Check sheet for the drawn part. Datum: minimum x, y, z corner. Units: mm. Round coordinates to 2 decimals unless told otherwise and drop trailing zeros. Write each loop counter-clockwise with the first axis right and the second up, starting at its lowest first coordinate (ties: lowest second). Pieces come first, ordered by that corner, then holes. Notation, with made-up numbers: (6.5, -24) -> (37.5, -24) arc R19 cw to (37.5, -19) -> close; hole circle Ø10 at (23.5, 36). An arc over 180 degrees is marked (long way). One line per item, written item: value.
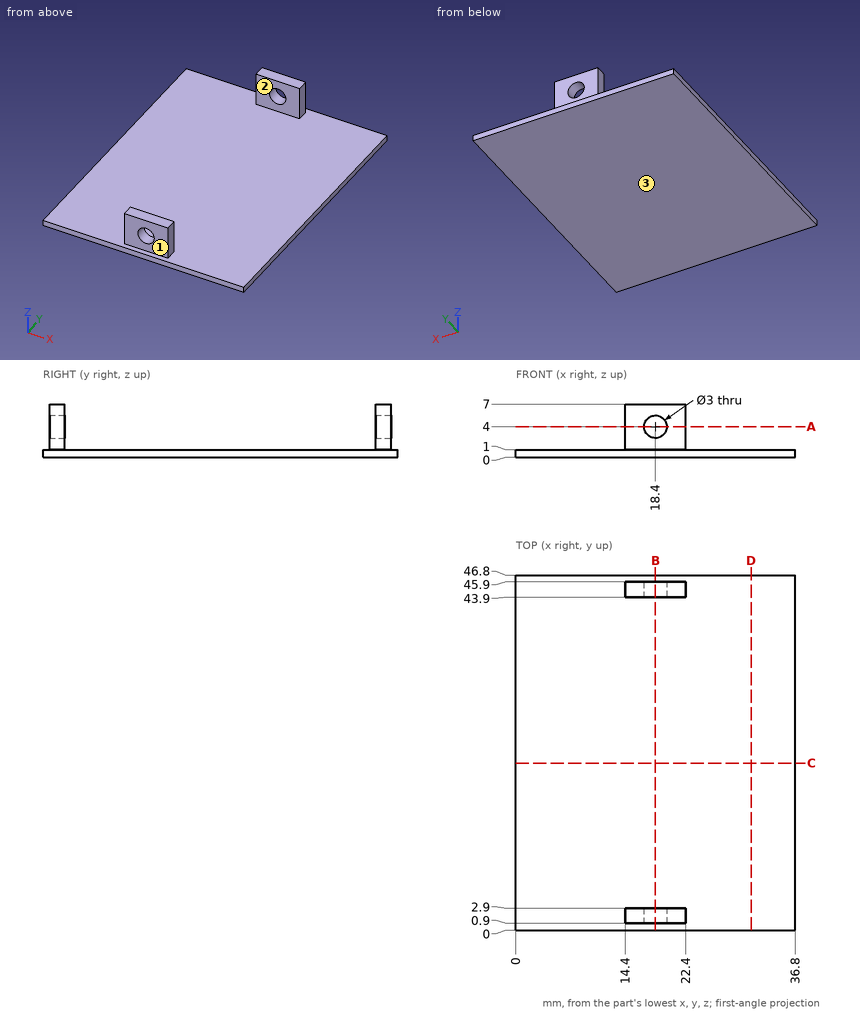
Item 1: Sectioned sample at B-B on x = 18.4. Enter the section's corners in (y, z), and give its area (3 significant figures).
Answer:
outline: (0, 0) -> (46.8, 0) -> (46.8, 1) -> (45.9, 1) -> (45.9, 2.5) -> (43.9, 2.5) -> (43.9, 1) -> (2.9, 1) -> (2.9, 2.5) -> (0.9, 2.5) -> (0.9, 1) -> (0, 1) -> close; (0.9, 5.5) -> (2.9, 5.5) -> (2.9, 7) -> (0.9, 7) -> close; (43.9, 5.5) -> (45.9, 5.5) -> (45.9, 7) -> (43.9, 7) -> close
area: 58.8 mm^2
Item 2: Sectioned sample at C-C on y = 22. Enter the section's corners in (x, z), and give its area (3 significant figures).
Answer:
outline: (0, 0) -> (36.8, 0) -> (36.8, 1) -> (0, 1) -> close
area: 36.8 mm^2
Item 3: Mould release check, pull along Y, two halves, no side actions. Record for the marked faces 1, 2 and 3: pulls with the +Y half, pulls with the -Y half, needs draft (parallel to the pull), parting line crosses it, or undercut.
Answer:
face 1: pulls with the -Y half
face 2: undercut
face 3: needs draft
Item 4: Depth check by flat-ended pin: P1, Ø11, axis at x = 13.5, y = 12, coming from the +Z side; P2, Ø1, axis at y = 2, z = 2.5, coming from the -X side; P3, Ø3, axis at x = 18, z = 4, coming from the -Y side. Enter the tip coordinate at first touch or a pass-through.
Answer:
P1: stops at z = 1
P2: stops at x = 14.4
P3: stops at y = 0.9
Item 5: Sectioned sample at A-A on z = 4. Enter the section's corners in (x, y), and give its area (3 significant figures).
Answer:
outline: (14.4, 0.9) -> (16.9, 0.9) -> (16.9, 2.9) -> (14.4, 2.9) -> close; (14.4, 43.9) -> (16.9, 43.9) -> (16.9, 45.9) -> (14.4, 45.9) -> close; (19.9, 0.9) -> (22.4, 0.9) -> (22.4, 2.9) -> (19.9, 2.9) -> close; (19.9, 43.9) -> (22.4, 43.9) -> (22.4, 45.9) -> (19.9, 45.9) -> close
area: 20.0 mm^2
Item 6: Sectioned sample at D-D on x = 31. Enter the section's corners in (y, z).
Answer:
outline: (0, 0) -> (46.8, 0) -> (46.8, 1) -> (0, 1) -> close
Item 7: Thickness scan on line 1 (Z direction, x = 18.4, y = 45.15); line 2 (Y direction, x = 16.5, z = 3); line 3 (X direction, y = 1.5, z = 4). Record the ranges inside material, lowest first.
Answer:
line 1: z = 0 to 2.5, 5.5 to 7
line 2: y = 0.9 to 2.9, 43.9 to 45.9
line 3: x = 14.4 to 16.9, 19.9 to 22.4
